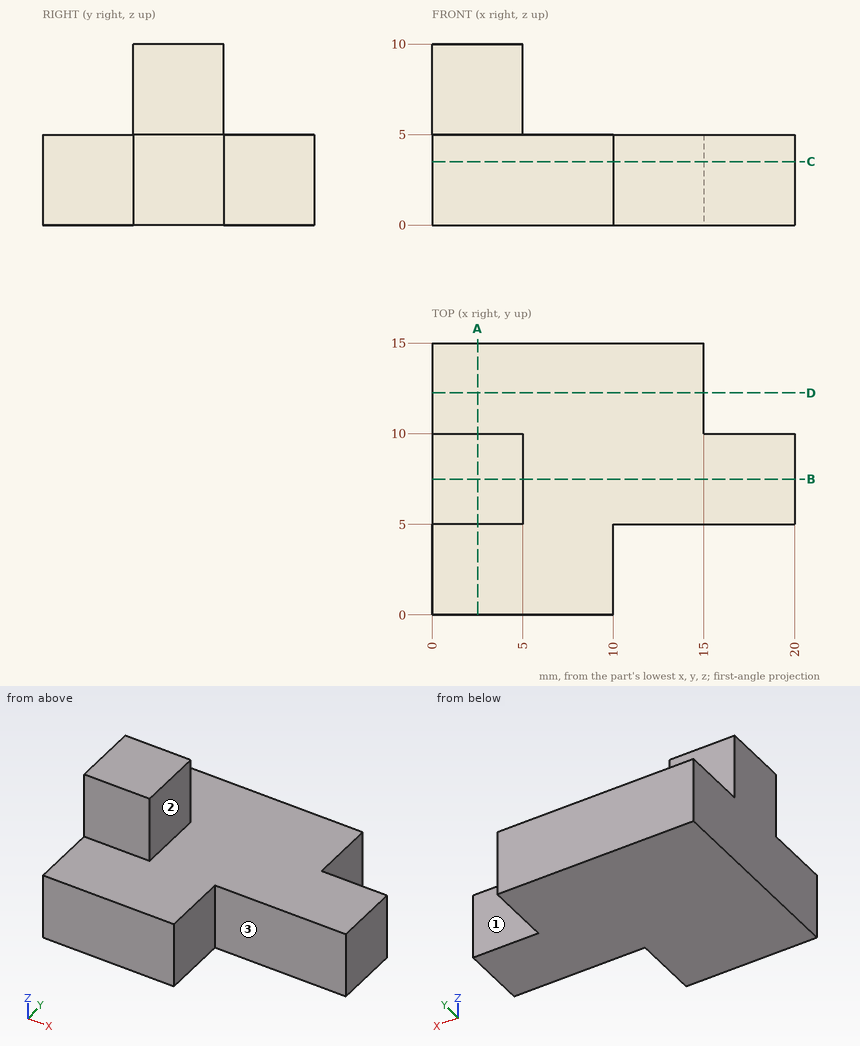
Geometry check sheet. Reference: drawing and pictorial views, mm from the part's lowest x, y, z. A direction names the side the tool comes from. Give positions to 0.01 mm unless a question says otherwise; leave off trailing zeros. Order: outer loops, then holes, each group sorted by start corner. A loop starts at its lowest first (then second) coordinate and runs counter-clockwise, first axis right, second up.
1. Section check D-D, the plane y = 12.25. Enter the section's corners in (x, z), and give its area (3 significant figures).
2. Gauge pin test, flat ends, axial feed: pin 1 Ø2 at (x, z) = (16.5, 5.5) entering from -Y; pin 2 Ø1.5 at (x, z) = (1.5, 8.5) entering from +Y; pin 3 Ø5 at (y, z) = (9.5, 8) entering from +X. Record the tip position at first contact, or that the pin passes through.
3. Access from +Z, -Z, +X, -X, +Y, -Y to the whole of each face (thin tool, end or side, straight path). Record for the marked faces 1, 2 and 3.
4. Section check C-C, the plane z = 3.5. Enter the section's corners in (x, y).
5. Section check A-A, the plane x = 2.5. Enter the section's corners in (y, z), and give its area (3 significant figures).
6. Thickness scan on L1, parallel to X at y = 6.25, z = 8.5; L2, parallel to X at y = 3, z = 3.25; L3, parallel to Y at x = 4, z = 6. Record the ranges inside material, lowest first.
7. Section check B-B, the plane y = 7.5. Enter the section's corners in (x, z), and give its area (3 significant figures).
Values follow:
1. outline: (0, 0) - (15, 0) - (15, 5) - (0, 5) - close
1. area: 75.0 mm2
2. pin 1: stops at y = 5
2. pin 2: stops at y = 10
2. pin 3: stops at x = 5
3. face 1: +Z, -Z, +X, +Y
3. face 2: +Z, +X, +Y, -Y
3. face 3: +Z, -Z, +X, -Y
4. outline: (0, 0) - (10, 0) - (10, 5) - (20, 5) - (20, 10) - (15, 10) - (15, 15) - (0, 15) - close
5. outline: (0, 0) - (15, 0) - (15, 5) - (10, 5) - (10, 10) - (5, 10) - (5, 5) - (0, 5) - close
5. area: 100 mm2
6. L1: x = 0 to 5
6. L2: x = 0 to 10
6. L3: y = 5 to 10
7. outline: (0, 0) - (20, 0) - (20, 5) - (5, 5) - (5, 10) - (0, 10) - close
7. area: 125 mm2
